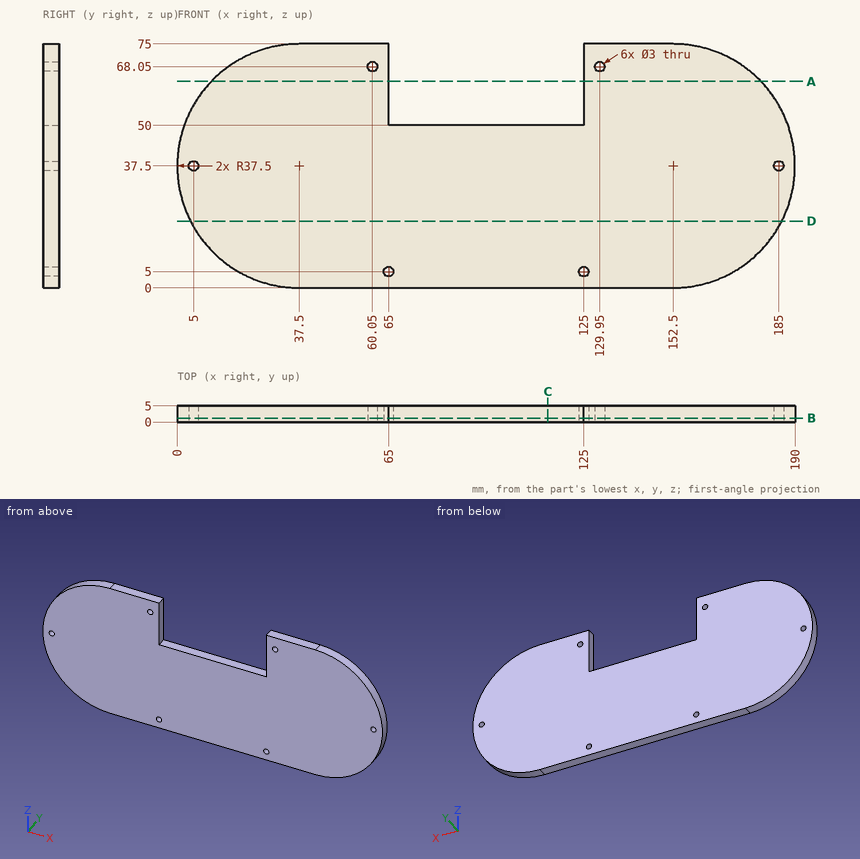
The drawing under review shows one solid part. Ordinate dimensions are in mm from its lowest x, y, z. Coordinates: 2 decimals unless noted, no trailing zeros. Write each loop counter-clockwise with the first axis right and the second up, starting at its lowest first coordinate (ties: lowest second). Pieces come first, ordered by that corner, then holes.
1) Add section D-D (z = 20.5). Write out the cut boundary in (x, y) (1 decimal).
2) To check wall thickness, follow L1, parallel to X at y = 3.4, z = 37.5; L2, parallel to X at y = 3.9, z = 5; L3, parallel to X at y = 4.35, z = 69 (1 decimal). State the ranges of each line that lie inside material, in increasing order.
3) Add section A-A (z = 63.5). Write out the cut boundary in (x, y), plus the area to 3 significant figures.
4) Add section C-C (x = 114). Write out the cut boundary in (y, z), plus the area to 3 significant figures.
5) Insertion check: pin 1 (1 mm diameter, centred on y = 2, z = 41, fed in from +X); pin 2 (1.5 mm diameter, centred on x = 163.5, y = 2.5, fed in from -Z); pin 3 (2 mm diameter, centred on x = 81.5, y = 4, fed in from +Z); pin 4 (4 mm diameter, centred on x = 60.05, z = 68.05, fed in from +Y). Each pin has a flat end and moves straight along its axis. Give the tip position at first contact, or say it passes through.
6) Add section B-B (y = 1.25). Write out the cut boundary in (x, z), plus the area to 3 significant figures.
Check result:
1. outline: (4.1, 0) - (185.9, 0) - (185.9, 5) - (4.1, 5) - close
2. L1: x = 0 to 3.5, 6.5 to 183.5, 186.5 to 190
2. L2: x = 18.79 to 63.5, 66.5 to 123.5, 126.5 to 171.21
2. L3: x = 17.2 to 58.9, 61.2 to 65, 125 to 128.8, 131.1 to 172.8
3. outline: (10.48, 0) - (65, 0) - (65, 5) - (10.48, 5) - close; (125, 0) - (179.52, 0) - (179.52, 5) - (125, 5) - close
3. area: 545 mm2
4. outline: (0, 0) - (5, 0) - (5, 50) - (0, 50) - close
4. area: 250 mm2
5. pin 1: stops at x = 189.88
5. pin 2: stops at z = 1.43
5. pin 3: stops at z = 50
5. pin 4: stops at y = 5
6. outline: (37.5, 0) - (152.5, 0) arc R37.5 ccw to (152.5, 75) - (125, 75) - (125, 50) - (65, 50) - (65, 75) - (37.5, 75) arc R37.5 ccw to start; hole circle Ø3 at (5, 37.5); hole circle Ø3 at (60.05, 68.05); hole circle Ø3 at (65, 5); hole circle Ø3 at (125, 5); hole circle Ø3 at (129.95, 68.05); hole circle Ø3 at (185, 37.5)
6. area: 11,500 mm2
